Design review of the part built by this model. Coordinates are the model's own, in mm. Face numbers are marked on the shaded views. A direction names the side the tool comes from. Coordinates: 2 decimals unless noted, no trailing zeros. Loops run counter-clockwise (first coordinate to the right, second up) from the corner with the lowest first, then second, coordinate; pieces in that order, holes last.
Autodesk Inventor part; units mm, degrees
ref_plane "YZ Plane" through (0, 0, 0) normal (1, 0, 0) x (0, 1, 0)
ref_plane "XZ Plane" through (0, 0, 0) normal (0, 1, 0) x (-1, 0, 0)
ref_plane "XY Plane" through (0, 0, 0) normal (0, 0, 1) x (1, 0, 0)
sketch "Sketch1" plane through (0, 0, 0) normal (0, 0, 1) x (1, 0, 0)
  line L0 (0, 0) -> (0, 200)
  line L1 (0, 200) -> (440, 200)
  line L2 (440, 200) -> (440, 0)
  line L3 (445, 0) -> (445, 205)
  line L4 (445, 205) -> (-5, 205)
  line L5 (-5, 205) -> (-5, 0)
  line L6 (-5, 0) -> (0, 0)
  line L7 (445, 0) -> (440, 0)
  dimension "d1" = 440
  dimension "d4" = 200
  dimension "d5" = 440
  dimension "d6" = 5
extrude "Extrusion1" add sketch "Sketch1" against normal blind 1655
properties part number "Proteção" material "Polycarbonate, Clear"
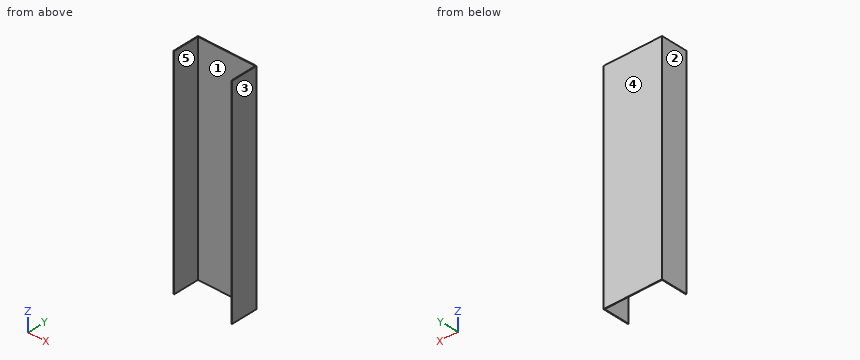
Q1. Take a section at B-B, the plane z = -616. Write out the cut boundary in (x, y), then the cut area to 3 significant figures.
Q2. The part is to be moulded in two halves that separate along X. For the marked faces 1, 2 and 3, say which applies: pulls with the +X half, pulls with the -X half, needs draft (parallel to the pull), parting line crosses it, or undercut.
Q3. Take a section at A-A, the plane y = 17. Write out the cut boundary in (x, z), then the cut area to 4 significant figures.
Q4. Take a section at C-C, the plane x = 388. Write out the cut boundary in (y, z), then the cut area to 4 significant figures.
Q5. Machinability: for the marked faces 4 and 5, which of the approach directions +Z, -Z, +X, -X, +Y, -Y give a long, thin tool a straight path to every point of the face, cutting with its end or side? Answer none if there is none.
Q6. For line 1 (X direction, y = 91.5, z = -1265.5); line 2 (Y direction, x = 118, z = -1355.5), list the stretches that pass through material, from the lowest coordinate up.
Q7. Clearance check with a flat-ended pin moving along its axis: pin 1 Ø1.5 at (x, z) = (143, -219.5) entering from -Y. State where the tip first meets the part, or that it passes through.
Entries:
1. outline: (-5, 0) - (0, 0) - (0, 200) - (440, 200) - (440, 0) - (445, 0) - (445, 205) - (-5, 205) - close
1. area: 4,250 mm2
2. face 1: undercut
2. face 2: pulls with the -X half
2. face 3: pulls with the +X half
3. outline: (-5, -1655) - (0, -1655) - (0, 0) - (-5, 0) - close; (440, -1655) - (445, -1655) - (445, 0) - (440, 0) - close
3. area: 16,550 mm2
4. outline: (200, -1655) - (205, -1655) - (205, 0) - (200, 0) - close
4. area: 8,275 mm2
5. face 4: +Z, -Z, +X, -X, +Y
5. face 5: +Z, -Z, -Y
6. line 1: x = -5 to 0, 440 to 445
6. line 2: y = 200 to 205
7. pin 1: stops at y = 200
